Autodesk Inventor part; units mm, degrees
ref_plane "YZ Plane" through (0, 0, 0) normal (1, 0, 0) x (0, 1, 0)
ref_plane "XZ Plane" through (0, 0, 0) normal (0, 1, 0) x (-1, 0, 0)
ref_plane "XY Plane" through (0, 0, 0) normal (0, 0, 1) x (1, 0, 0)
sketch "Sketch1" plane through (0, 0, 0) normal (0, 1, 0) x (-1, 0, 0)
  line L0 (0, 0) -> (-584.2, 0)
  line L1 (-584.2, 0) -> (-584.2, -812.8)
  line L2 (-584.2, -812.8) -> (0, -812.8)
  line L3 (0, -812.8) -> (0, 0)
  dimension "d0" = 584.2
  dimension "d1" = 812.8
extrude "Extrusion1" add sketch "Sketch1" along normal blind 3.175
sketch "Sketch2" plane through (0, 0, 0) normal (0, -1, 0) x (1, 0, 0)
  line L0 (0, 0) -> (584.2, 0)
  line L1 (0, -812.8) -> (0, 0)
  line L2 (584.2, -812.8) -> (0, -812.8)
  line L3 (584.2, 0) -> (584.2, -812.8)
  line L4 (584.2, 0) -> (584.2, -812.8)
  line L5 (584.2, -323.85) -> (558.8, -323.85)
  line L6 (558.8, -323.85) -> (558.8, -488.95)
  line L7 (558.8, -488.95) -> (584.2, -488.95)
  line L8 (584.2, -488.95) -> (584.2, -323.85)
  line L9 (0, -812.8) -> (0, 0)
  line L10 (0, -323.85) -> (25.4, -323.85)
  line L11 (25.4, -323.85) -> (25.4, -488.95)
  line L12 (25.4, -488.95) -> (0, -488.95)
  line L13 (0, -488.95) -> (0, -323.85)
  line L14 (584.2, 0) -> (508, 0)
  line L15 (508, 0) -> (508, -228.6)
  line L16 (508, -228.6) -> (584.2, -228.6)
  line L17 (584.2, -228.6) -> (584.2, 0)
  line L18 (0, 0) -> (76.2, 0)
  line L19 (76.2, 0) -> (76.2, -228.6)
  line L20 (76.2, -228.6) -> (0, -228.6)
  line L21 (0, -228.6) -> (0, 0)
  line L22 (0, -812.8) -> (76.2, -812.8)
  line L23 (76.2, -812.8) -> (76.2, -584.2)
  line L24 (76.2, -584.2) -> (0, -584.2)
  line L25 (0, -584.2) -> (0, -812.8)
  line L26 (584.2, -812.8) -> (508, -812.8)
  line L27 (508, -812.8) -> (508, -584.2)
  line L28 (508, -584.2) -> (584.2, -584.2)
  line L29 (584.2, -584.2) -> (584.2, -812.8)
  line L30 (508, -228.6) -> (393.7, -228.6)
  line L31 (393.7, -228.6) -> (393.7, -152.4)
  line L32 (393.7, -152.4) -> (508, -152.4)
  line L33 (508, -152.4) -> (508, -228.6)
  line L34 (508, -584.2) -> (393.7, -584.2)
  line L35 (393.7, -584.2) -> (393.7, -660.4)
  line L36 (393.7, -660.4) -> (508, -660.4)
  line L37 (508, -660.4) -> (508, -584.2)
  line L38 (76.2, -584.2) -> (190.5, -584.2)
  line L39 (190.5, -584.2) -> (190.5, -660.4)
  line L40 (190.5, -660.4) -> (76.2, -660.4)
  line L41 (76.2, -660.4) -> (76.2, -584.2)
  line L42 (76.2, -228.6) -> (190.5, -228.6)
  line L43 (190.5, -228.6) -> (190.5, -152.4)
  line L44 (190.5, -152.4) -> (76.2, -152.4)
  line L45 (76.2, -152.4) -> (76.2, -228.6)
  dimension "d4" = 165.1
  dimension "d5" = 165.1
  dimension "d6" = 25.4
  dimension "d7" = 25.4
  dimension "d8" = 323.85
  dimension "d9" = 323.85
  dimension "d10" = 76.2
  dimension "d11" = 228.6
  dimension "d12" = 76.2
  dimension "d13" = 228.6
  dimension "d14" = 76.2
  dimension "d15" = 228.6
  dimension "d16" = 76.2
  dimension "d17" = 228.6
  dimension "d18" = 114.3
  dimension "d19" = 76.2
  dimension "d20" = 114.3
  dimension "d21" = 76.2
  dimension "d22" = 114.3
  dimension "d23" = 76.2
  dimension "d24" = 114.3
  dimension "d25" = 76.2
extrude "Extrusion2" cut sketch "Sketch2" against normal blind 3.175 contours L0 L19 L20 L1 | L0 L3 L16 L15 | L44 L43 L42 L19 | L10 L11 L12 L1 | L15 L30 L31 L32 | L24 L23 L2 L1 | L3 L7 L6 L5 | L38 L39 L40 L23 | L3 L2 L27 L28 | L27 L36 L35 L34
properties part number "polycarb base" material "Polycarbonate, Clear"
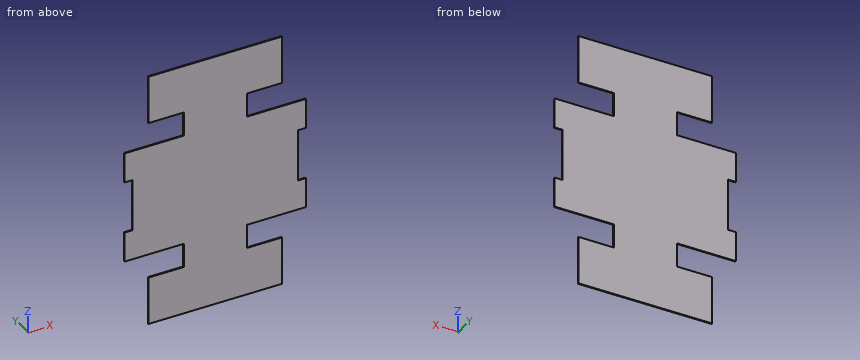
For this review, take the finished solid that the model builds, in its own axes (mm). Give positions to 0.01 mm unless a question says otherwise; leave off trailing zeros. Order: outer loops, then holes, each group sorted by start corner. A loop starts at its lowest first (then second) coordinate and runs counter-clockwise, first axis right, second up. Notation, with made-up numbers: M -7,5 L 2,5 A9 cw 2,14 Z; hole C -37,-29.5 d10. An arc over 180 degrees is marked long. Answer in a Markdown table with one row per item. Add a question column.
(1) Wall thickness on probe 1 along Z at (x, y) = (498, 2.65); probe 2 along Z at (x, y) = (542.5, 1.45); probe 3 along X at (y, z) = (0.6, -38.5): over which ranges is each line inside the solid? List them lowest first. Write a range as [from, to].
(2) Consider section A-A on x = 433. State the section outline as (y, z) points (3 decimals).
(3) Consider section C-C on z = -606. State the section outline as (x, y) points (3 decimals).
(4) Consider section B-B on y = 0.9. State the section outline as (x, z) points.
(5) For pin 1 (1.6 mm diameter, centred on y = 2, z = -724, fed in from +X); pin 2 (1.6 mm diameter, centred on y = 1.5, z = -379.5, fed in from +X); pin 3 (1.6 mm diameter, centred on x = 70, y = 1.5, fed in from -Z), all flat-tipped, find the tip position at first contact; note any pin that passes through.
(6) Consider section D-D on x = 66.5. State the section outline as (y, z) points (3 decimals).
Evaluation:
| question | item | result |
|---|---|---|
| 1 | probe 1 | z = [-812.8, -660.4], [-584.2, -228.6], [-152.4, 0] |
| 1 | probe 2 | z = [-584.2, -228.6] |
| 1 | probe 3 | x = [76.2, 508] |
| 2 | outline | M 0,-812.8 L 3.175,-812.8 L 3.175,-660.4 L 0,-660.4 Z; M 0,-584.2 L 3.175,-584.2 L 3.175,-228.6 L 0,-228.6 Z; M 0,-152.4 L 3.175,-152.4 L 3.175,0 L 0,0 Z |
| 3 | outline | M 190.5,0 L 393.7,0 L 393.7,3.175 L 190.5,3.175 Z |
| 4 | outline | M 0,-584.2 L 190.5,-584.2 L 190.5,-660.4 L 76.2,-660.4 L 76.2,-812.8 L 508,-812.8 L 508,-660.4 L 393.7,-660.4 L 393.7,-584.2 L 584.2,-584.2 L 584.2,-488.95 L 558.8,-488.95 L 558.8,-323.85 L 584.2,-323.85 L 584.2,-228.6 L 393.7,-228.6 L 393.7,-152.4 L 508,-152.4 L 508,0 L 76.2,0 L 76.2,-152.4 L 190.5,-152.4 L 190.5,-228.6 L 0,-228.6 L 0,-323.85 L 25.4,-323.85 L 25.4,-488.95 L 0,-488.95 Z |
| 5 | pin 1 | stops at x = 508 |
| 5 | pin 2 | stops at x = 558.8 |
| 5 | pin 3 | stops at z = -584.2 |
| 6 | outline | M 0,-584.2 L 3.175,-584.2 L 3.175,-228.6 L 0,-228.6 Z |
